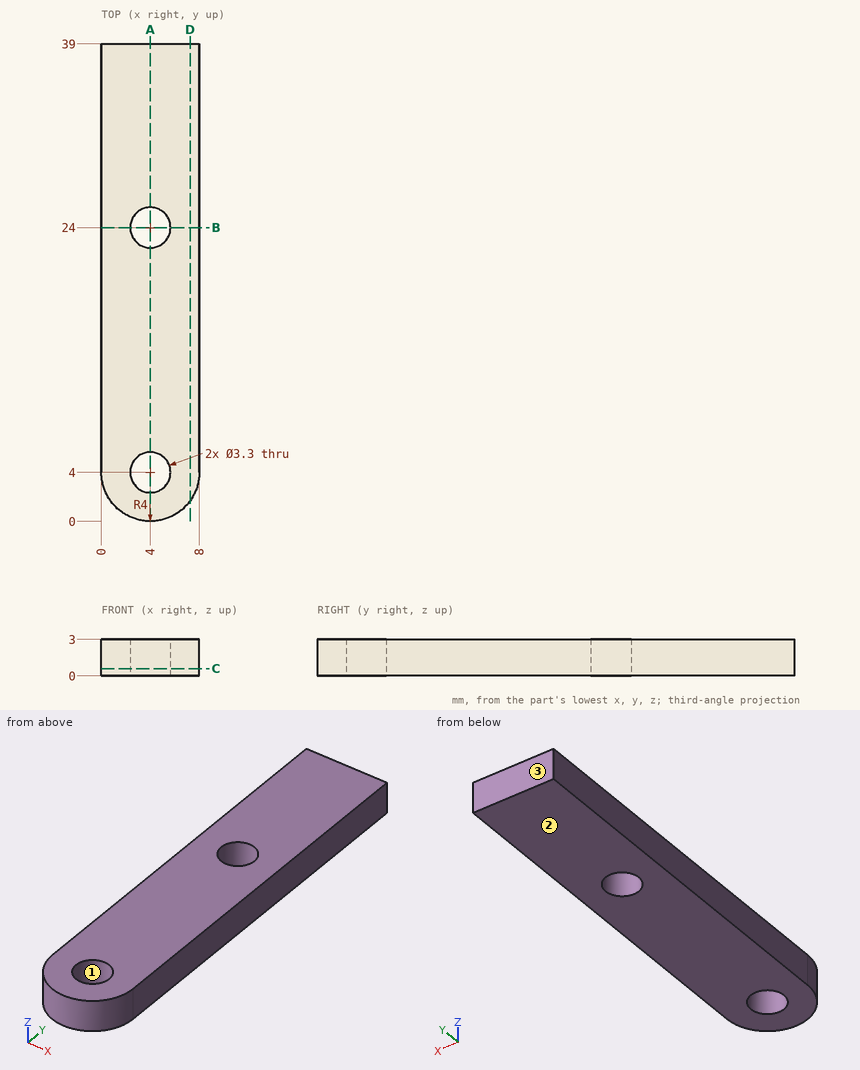
Check sheet for the drawn part. Datum: minimum x, y, z corner. Units: mm. Give positions to 0.01 mm unless a question says otherwise; leave off trailing zeros. Write each loop counter-clockwise with the first axis right and the second up, starting at its lowest first coordinate (ties: lowest second). Pieces come first, ordered by that corner, then holes. Notation, with made-up numbers: M -18,39 L 16,39 A22 cw 16,65 Z; hole C 7,82 d4. An arc over 180 degrees is marked long. Write item = value, one per line.
(1) Sectioned sample at C-C (z = 0.6). Record the cut outline in (x, y), then the cut area to 3 significant figures.
Found:
outline = M 0,4 A4 ccw 8,4 L 8,39 L 0,39 Z; hole C 4,4 d3.3; hole C 4,24 d3.3
area = 288 mm2
(2) Material ranges on line 1 (Y direction, x = 4, z = 1.85); line 2 (Y direction, x = 2.5, z = 1.6); line 3 (Y direction, x = 1.5, z = 2.7), recorded low to high.
Found:
line_1 = 0 to 2.35, 5.65 to 22.35, 25.65 to 39
line_2 = 0.29 to 3.31, 4.69 to 23.31, 24.69 to 39
line_3 = 0.88 to 39
(3) Sectioned sample at B-B (y = 24). Record the cut outline in (x, z).
Found:
outline = M 0,0 L 2.35,0 L 2.35,3 L 0,3 Z; M 5.65,0 L 8,0 L 8,3 L 5.65,3 Z
(4) Sectioned sample at A-A (x = 4). Record the cut outline in (y, z).
Found:
outline = M 0,0 L 2.35,0 L 2.35,3 L 0,3 Z; M 5.65,0 L 22.35,0 L 22.35,3 L 5.65,3 Z; M 25.65,0 L 39,0 L 39,3 L 25.65,3 Z
(5) Draft check along Y on the marked faces 1, 2 and 3. Enter one of: released by +Y, released by -Y, zero draft, split by the parting line, or undercut.
Found:
face_1 = undercut
face_2 = zero draft
face_3 = released by +Y
(6) Sectioned sample at D-D (x = 7.25). Record the cut outline in (y, z), then the cut area to 3 significant figures.
Found:
outline = M 1.67,0 L 39,0 L 39,3 L 1.67,3 Z
area = 112 mm2
